Check sheet for the modelled part. Datum: model origin and axes. Units: mm. Round coordinates to 2 decimals unless told otherwise and drop trailing zeros. Write each loop counter-clockwise with the first axis right and the second up, starting at its lowest first coordinate (ties: lowest second). Pieces come first, ordered by that corner, then holes. Notation, with made-up numbers: (12.5, 27) -> (16.5, 27) arc R32 cw to (16.5, 54) -> close; hole circle Ø2 at (58.25, 59). An arc over 180 degrees is marked (long way). Write item = value, one per line.
from build123d import *

# Parameters (mm, degrees)
SKETCH_1_W          = 10
SKETCH_1_H          = 20
SKETCH_1_W_2        = 7.6
SKETCH_1_H_2        = 17.6
EXTRUDE_1_DEPTH     = 660
SKETCH_2_R          = 2
CUT_EXTRUDE_1_DEPTH = 661.321891202
SKETCH_3_R          = 1.5
SKETCH_3_R_2        = 2
CUT_EXTRUDE_2_DEPTH = 661.151497764


with BuildPart() as part:
    # ｽｹｯﾁ1 → 押し出し-薄板1 (new body)
    with BuildSketch(Plane(origin=(0, 0, 0), x_dir=(0, 0, -1), z_dir=(1, 0, 0))):
        Rectangle(SKETCH_1_W, SKETCH_1_H)
        Rectangle(SKETCH_1_W_2, SKETCH_1_H_2, mode=Mode.SUBTRACT)
    extrude(amount=EXTRUDE_1_DEPTH)

    # ｽｹｯﾁ2 → ｶｯﾄ - 押し出し1 (cut, through all)
    with BuildSketch(Plane(origin=(0, 10, 0), x_dir=(1, 0, 0), z_dir=(0, 1, 0))):
        with Locations(Location((5, 0, 0), (0, 0, 270))):
            Circle(SKETCH_2_R)
        with Locations(Location((70, 0, 0), (0, 0, 270))):
            Circle(SKETCH_2_R)
        with Locations(Location((135, 0, 0), (0, 0, 270))):
            Circle(SKETCH_2_R)
        with Locations(Location((525, 0, 0), (0, 0, 270))):
            Circle(SKETCH_2_R)
        with Locations(Location((590, 0, 0), (0, 0, 270))):
            Circle(SKETCH_2_R)
        with Locations(Location((655, 0, 0), (0, 0, 270))):
            Circle(SKETCH_2_R)
        with Locations(Location((199, 0, 0), (0, 0, 270))):
            Circle(SKETCH_2_R)
        with Locations(Location((179, 0, 0), (0, 0, 270))):
            Circle(SKETCH_2_R)
        with Locations(Location((481, 0, 0), (0, 0, 270))):
            Circle(SKETCH_2_R)
        with Locations(Location((461, 0, 0), (0, 0, 270))):
            Circle(SKETCH_2_R)
        with Locations(Location((357.5, 0, 0), (0, 0, 270))):
            Circle(SKETCH_2_R)
        with Locations(Location((302.5, 0, 0), (0, 0, 270))):
            Circle(SKETCH_2_R)
    extrude(amount=-CUT_EXTRUDE_1_DEPTH, mode=Mode.SUBTRACT)

    # ｽｹｯﾁ3 → ｶｯﾄ - 押し出し2 (cut, through all)
    with BuildSketch(Plane.XY.offset(5)):
        with Locations((347.5, 0)):
            Circle(SKETCH_3_R)
        with Locations(Location((312.5, 0, 0), (0, 0, 90))):
            Circle(SKETCH_3_R)
        with Locations((342.5, 5)):
            Circle(SKETCH_3_R_2)
        with Locations(Location((342.5, -5, 0), (0, 0, 90))):
            Circle(SKETCH_3_R_2)
        with Locations((317.5, -5)):
            Circle(SKETCH_3_R_2)
        with Locations(Location((317.5, 5, 0), (0, 0, 90))):
            Circle(SKETCH_3_R_2)
        with Locations((15, 0)):
            Circle(SKETCH_3_R_2)
        with Locations((35, 0)):
            Circle(SKETCH_3_R_2)
        with Locations((55, 0)):
            Circle(SKETCH_3_R_2)
        with Locations(Location((605, 0, 0), (0, 0, 90))):
            Circle(SKETCH_3_R_2)
        with Locations(Location((625, 0, 0), (0, 0, 90))):
            Circle(SKETCH_3_R_2)
        with Locations(Location((645, 0, 0), (0, 0, 90))):
            Circle(SKETCH_3_R_2)
    extrude(amount=-CUT_EXTRUDE_2_DEPTH, mode=Mode.SUBTRACT)


solid = part.part
(1) Sectioned sample at B-B on z = 0. Count the separate pieces of the cut face and the enclosed holes in it, then the cut area to 3 significant figures.
Worked answers:
separate_pieces = 26
enclosed_holes = 0
area = 1,470 mm²
(2) Material ranges on L1, parallel to Y at x = 242, z = -0.75; L2, parallel to Z at x = 429.5, y = 2; L3, parallel to Z at x = 179, y = 9.35, recorded low to high. Write a range as [from, to].
Worked answers:
L1 = [-10, -8.8], [8.8, 10]
L2 = [-5, -3.8], [3.8, 5]
L3 = [-5, -2], [2, 5]
(3) Go/stop test with flat-tipped pins: P1, Ø3.5, axis at x = 357.5, z = 0, coming from the -Y side; P2, Ø5, axis at x = 655, z = 0, coming from the -Y side. Record where each tip stops, or that it passes through.
Worked answers:
P1 = through
P2 = -10
(4) Sectioned sample at A-A on x = 275. Enter the section's corners in (y, z).
Worked answers:
outline = (-10, -5) -> (10, -5) -> (10, 5) -> (-10, 5) -> close; hole (-8.8, -3.8) -> (8.8, -3.8) -> (8.8, 3.8) -> (-8.8, 3.8) -> close
(5) Release check for a two-part mould opening along Z. For faces 1 (the flat face through (325, 0, -5)), 2 (the flat face through (0, -1, 4)), 3 (the flat face through (325, 0, -3.8)), 4 (the flat face through (325, 0, 3.8)) record: pulls with the +Z half, pulls with the -Z half, needs draft (parallel to the pull), parting line crosses it, or undercut.
Worked answers:
face_1 = pulls with the -Z half
face_2 = needs draft
face_3 = undercut
face_4 = undercut
